Geometry check sheet. Reference: the model listing, model coordinates, mm. A direction names the side the tool comes from. Give positions to 0.01 mm unless a question says otherwise; leave off trailing zeros. Order: outer loops, then holes, each group sorted by start corner. A loop starts at its lowest first (then second) coordinate and runs counter-clockwise, first axis right, second up.
from build123d import *

# Parameters (mm, degrees)
FILLET1_R = 3.175


with BuildPart() as part:
    # Sketch1 → Revolve1 (revolve)
    with BuildSketch(Plane(origin=(0, 0, 0), x_dir=(0, 0, -1), z_dir=(1, 0, 0)), mode=Mode.PRIVATE) as revolve1_sk:
        Polygon((0, 26.9875), (0, 0), (3.175, 0), (3.175, 23.8125), (155.575, 23.8125), (155.575, 25.7175), (158.75, 25.7175), (158.75, 19.05), (152.4, 19.05), (152.4, 0), (155.575, 0), (155.575, 15.875), (161.925, 15.875), (161.925, 28.8925), (152.4, 28.8925), (152.4, 26.9875), align=None)
    revolve(revolve1_sk.sketch.rotate(Axis((0, 0, 0), (0, 0, -1)), 90), axis=Axis((0, 0, 0), (0, 0, -1)))

    # Fillet1
    fillet1_edges = [part.edges().sort_by_distance(p)[0] for p in [
        (-26.9875, 0, 0),
    ]]
    fillet(fillet1_edges, radius=FILLET1_R)


solid = part.part
Item 1: Scan lines: L1, parallel to Z at x = -11, y = 18 (3 decimals); L2, parallel to Y at x = 0, z = -105; L3, parallel to Z at x = -3.5, y = 15 (3 decimals). Record each from-to range of solid material in increasing order.
Reported:
L1: z = -161.925 to -158.75, -3.175 to 0
L2: y = -26.99 to -23.81, 23.81 to 26.99
L3: z = -155.575 to -152.4, -3.175 to 0
Item 2: Draft check along X on faces 1 (the flat face through (0, 0, -3.175)), 2 (the flat face through (-24, -13, -152.4)), 3 (the cylindrical face through (-19.89, -18.24, -76.74)). Enter one of: released by +X, released by -X, zero draft, split by the parting line, or undercut.
Reported:
face 1: undercut
face 2: zero draft
face 3: split by the parting line
Item 3: Sectioned sample at C-C (z = -131.5). Enter the section's corners in (x, y) (1 decimal).
Reported:
outline: circle Ø54 at (0, 0); hole circle Ø47.6 at (0, 0)
Item 4: Gauge pin test, flat ends, axial feed: pin 1 (1 mm diameter, centred on x = -3, z = -26, fed in from +Y); pin 2 (1.5 mm diameter, centred on y = -2.5, z = -21.5, fed in from +X); pin 3 (1.5 mm diameter, centred on y = 17, z = -122.5, fed in from -X). Record the tip position at first contact, or that the pin passes through.
Reported:
pin 1: stops at y = 26.87
pin 2: stops at x = 26.93
pin 3: stops at x = -21.55
Item 5: Set-up check for faces 4 (the flat face through (0, 0, -155.575)), 5 (the flat face through (0, 0, -152.4)), 6 (the cylindrical face through (-6.263, 28.205, -157.096)): record each of +Z, -Z, +X, -X, +Y, -Y from which the full face is reachable in a straight line by a thin tool's end or side.
Reported:
face 4: -Z
face 5: none
face 6: +Z, -Z
